Build history of the part. All positions in model axes, mm. A direction names the side the tool comes from. Give positions to 0.01 mm unless a question says otherwise; leave off trailing zeros. Order: outer loops, then holes, each group sorted by start corner. A loop starts at its lowest first (then second) coordinate and runs counter-clockwise, first axis right, second up. Notation, with made-up numbers: (4, 76) - (39, 76) arc R14 ccw to (39, 80) - close; hole circle Ø10 at (30.5, -20). An arc over 180 degrees is marked (long way). Answer in a Markdown table with one row per item.
```python
from build123d import *

# Parameters (mm, degrees)
SCHNITT_LINEAR_AUSTRAGEN1_DEPTH = 4


with BuildPart() as part:
    # Skizze1 → Rotation1 (revolve)
    with BuildSketch(Plane(origin=(0, 0, 0), x_dir=(0, 0, -1), z_dir=(1, 0, 0)), mode=Mode.PRIVATE) as rotation1_sk:
        Polygon((-5, 0), (-5, 3), (162.3, 3), (162.3, 6), (165.3, 6), (165.3, 0), align=None)
    revolve(rotation1_sk.sketch.rotate(Axis((0, 0, -165.3), (0, 0, 1)), 270), axis=Axis((0, 0, -165.3), (0, 0, 1)))

    # Skizze2 → Rotation2 (revolve)
    with BuildSketch(Plane(origin=(0, 0, 0), x_dir=(0, 0, -1), z_dir=(1, 0, 0)), mode=Mode.PRIVATE) as rotation2_sk:
        with BuildLine():
            Line((-21, 0), (-21, 2.3865))
            Line((-21, 2.3865), (-20.3865, 3))
            Line((-20.3865, 3), (-8.148486452, 3))
            Line((-8.148486452, 3), (-6.599415898, 2.436184428))
            ThreePointArc((-6.599415898, 2.436184428), (-6.498392718, 2.409115348), (-6.394203812, 2.4))
            Line((-6.394203812, 2.4), (-5.6, 2.4))
            ThreePointArc((-5.6, 2.4), (-5.175735931, 2.575735931), (-5, 3))
            Line((-5, 3), (-4, 3))
            Line((-4, 3), (-4, 0))
            Line((-4, 0), (-21, 0))
        make_face()
    revolve(rotation2_sk.sketch.rotate(Axis((0, 0, 4), (0, 0, 1)), 270), axis=Axis((0, 0, 4), (0, 0, 1)))

    # Skizze3 → Schnitt-Linear austragen1 (cut)
    with BuildSketch(Plane.XY.offset(2)):
        Polygon((-5, 10), (-5, -5), (-2.5, -5), (-2.5, 5), (2.5, 5), (2.5, -5), (5, -5), (5, 10), align=None)
    extrude(amount=SCHNITT_LINEAR_AUSTRAGEN1_DEPTH, mode=Mode.SUBTRACT)


solid = part.part
```
1. Cut at B-B on y = 0. Write the cut outline in (x, z).
Check result:
| item | result |
|---|---|
| outline | (-6, -165.3) - (6, -165.3) - (6, -162.3) - (3, -162.3) - (3, 2) - (2.5, 2) - (2.5, 5.27) arc R0.6 cw to (2.4, 5.6) - (2.4, 6.39) arc R0.6 cw to (2.44, 6.6) - (3, 8.15) - (3, 20.39) - (2.39, 21) - (-2.39, 21) - (-3, 20.39) - (-3, 8.15) - (-2.44, 6.6) arc R0.6 cw to (-2.4, 6.39) - (-2.4, 5.6) arc R0.6 cw to (-2.5, 5.27) - (-2.5, 2) - (-3, 2) - (-3, -162.3) - (-6, -162.3) - close |
2. Cut at A-A on x = 0. Write the cut outline in (y, z).
Check result:
| item | result |
|---|---|
| outline | (-6, -165.3) - (6, -165.3) - (6, -162.3) - (3, -162.3) - (3, 5) arc R0.6 cw to (2.4, 5.6) - (2.4, 6.39) arc R0.6 cw to (2.44, 6.6) - (3, 8.15) - (3, 20.39) - (2.39, 21) - (-2.39, 21) - (-3, 20.39) - (-3, 8.15) - (-2.44, 6.6) arc R0.6 cw to (-2.4, 6.39) - (-2.4, 5.6) arc R0.6 cw to (-3, 5) - (-3, -162.3) - (-6, -162.3) - close |
3. Two-plate mould, pull along Z, no slides. Class faces 4 (the face through (5.723, 1.802, -163.821)), 5 (the face through (0, 0, -165.3)), 6 (the face through (1.29, 2.024, 5.992)), 7 (the face through (0, 0, 21)): +Z half, -Z half, draft (parallel to the pull), parting line (faces both ways), or undercut.
Check result:
| item | result |
|---|---|
| face 4 | draft |
| face 5 | -Z half |
| face 6 | undercut |
| face 7 | +Z half |
4. Drop flat-ended pins along their axis: P1, Ø1, axis at y = 0, z = 3.5, coming from the -X side; P2, Ø1.6, axis at y = 0, z = 4, coming from the +X side; P3, Ø1, axis at x = -2.5, z = -131.5, coming from the -Y side; P4, Ø6, axis at x = 1.5, y = -3, coming from the +Z side. Give the stop position or say it passes through.
Check result:
| item | result |
|---|---|
| P1 | stops at x = -2.5 |
| P2 | stops at x = 2.5 |
| P3 | stops at y = -2.24 |
| P4 | stops at z = 21 |
5. Probe line 1 (Z direction, x = -0.25, y = 3.25); line 2 (X direction, y = -2.5, z = -142). List the from-to ranges inside material, lowest first.
Check result:
| item | result |
|---|---|
| line 1 | z = -165.3 to -162.3 |
| line 2 | x = -1.66 to 1.66 |
6. Which spindle directions (+Z, -Z, +X, -X, +Y, -Y) get a long thin tool onto all of the face, cutting with end or side? Do faces 1 (the face through (-2.5, 0, 4)), 2 (the face through (3, -1, -162.3)), 3 (the face through (2.5, 0, 4)). Say none if no direction does.
Check result:
| item | result |
|---|---|
| face 1 | -X, +Y, -Y |
| face 2 | +Z |
| face 3 | +X, +Y, -Y |
7. Cut at C-C on z = -79. Write the cut outline in (x, y), and give its area (3 significant figures).
Check result:
| item | result |
|---|---|
| outline | circle Ø6 at (0, 0) |
| area | 28.3 mm² |
